Geometry check sheet. Reference: drawing and pictorial views, mm from the part's lowest x, y, z. A direction names the side the tool comes from. Round coordinates to 2 decimals unless told otherwise and drop trailing zeros. Loops run counter-clockwise (first coordinate to the right, second up) from the corner with the lowest first, then second, coordinate; pieces in that order, holes last. Notation, with made-up numbers: (62, 7.5) - (100, 7.5) arc R9 cw to (100, 12.5) - close; hole circle Ø10 at (-10.5, 74). An arc over 180 degrees is marked (long way). Return JSON: item names as keys, results as strings.
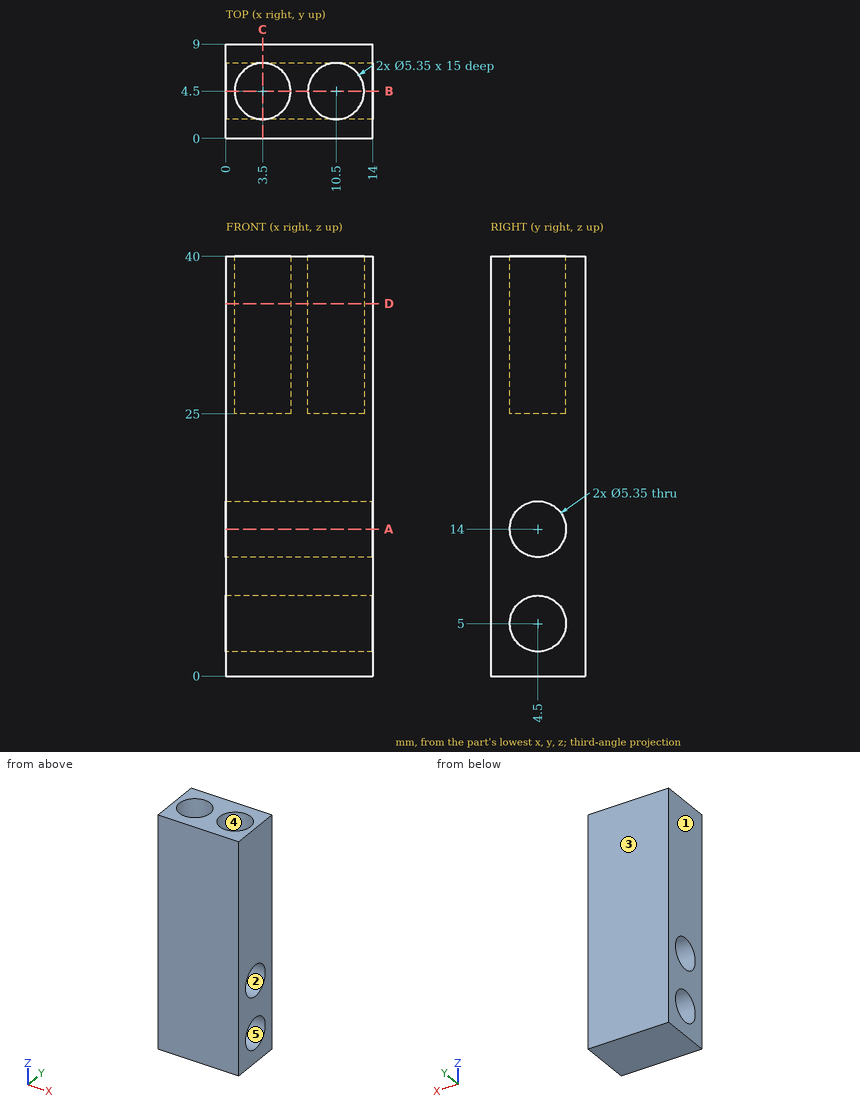
Q1. Sectioned sample at A-A (z = 14). Enter the section's corners in (x, y) (3 decimals), plus the area to 3 significant figures.
Answer key:
{"outline": "(0, 0) - (14, 0) - (14, 1.825) - (0, 1.825) - close; (0, 7.175) - (14, 7.175) - (14, 9) - (0, 9) - close", "area": "51.1 mm²"}
Q2. Depth check by flat-ended pin: P1, Ø2.5, axis at x = 3, y = 5, coming from the +Z side. Enter the tip coordinate at first touch or a pass-through.
Answer key:
{"P1": "stops at z = 25"}
Q3. Draft check along Y on the marked faces 1, 2 and 3. Enter one of: released by +Y, released by -Y, zero draft, split by the parting line, or undercut.
Answer key:
{"face 1": "zero draft", "face 2": "undercut", "face 3": "released by +Y"}
Q4. Tool access check on the marked faces 4 and 5. Record the directions out of +Z, -Z, +X, -X, +Y, -Y that give a thin tool (end or side, any length) a straight path to the whole face; none if there is none.
Answer key:
{"face 4": "+Z", "face 5": "+X, -X"}
Q5. Scan lines: probe 1 along Z at (x, y) = (8, 5.75); probe 2 along X at (y, z) = (4.75, 32); probe 3 along Y at (x, z) = (10.25, 14) (3 decimals). Record each from-to range of solid material in increasing order. Write a range as [from, to].
Answer key:
{"probe 1": "z = [0, 2.64], [7.36, 11.64], [16.36, 40]", "probe 2": "x = [0, 0.84], [6.16, 7.84], [13.16, 14]", "probe 3": "y = [0, 1.825], [7.175, 9]"}
Q6. Sectioned sample at D-D (z = 35.5). Enter the section's corners in (x, y) (3 decimals).
Answer key:
{"outline": "(0, 0) - (14, 0) - (14, 9) - (0, 9) - close; hole circle Ø5.35 at (3.5, 4.5); hole circle Ø5.35 at (10.5, 4.5)"}
Q7. Sectioned sample at C-C (x = 3.5). Enter the section's corners in (y, z) (3 decimals).
Answer key:
{"outline": "(0, 0) - (9, 0) - (9, 40) - (7.175, 40) - (7.175, 25) - (1.825, 25) - (1.825, 40) - (0, 40) - close; hole circle Ø5.35 at (4.5, 5); hole circle Ø5.35 at (4.5, 14)"}
Q8. Sectioned sample at B-B (y = 4.5). Enter the section's corners in (x, z) (3 decimals).
Answer key:
{"outline": "(0, 0) - (14, 0) - (14, 2.325) - (0, 2.325) - close; (0, 7.675) - (14, 7.675) - (14, 11.325) - (0, 11.325) - close; (0, 16.675) - (14, 16.675) - (14, 40) - (13.175, 40) - (13.175, 25) - (7.825, 25) - (7.825, 40) - (6.175, 40) - (6.175, 25) - (0.825, 25) - (0.825, 40) - (0, 40) - close"}
